Build history of the part. All positions in model axes, mm. Give positions to 0.01 mm unless a question says otherwise; leave off trailing zeros. Order: outer loops, then holes, each group sorted by start corner. A loop starts at its lowest first (then second) coordinate and runs counter-clockwise, first axis right, second up. Notation, with made-up numbers: M 9,29.25 L 36,29.25 A16 ccw 36,47.25 Z; hole C 19.5,31 d4. An arc over 180 degrees is marked long. Answer as CSV lines item,"result".
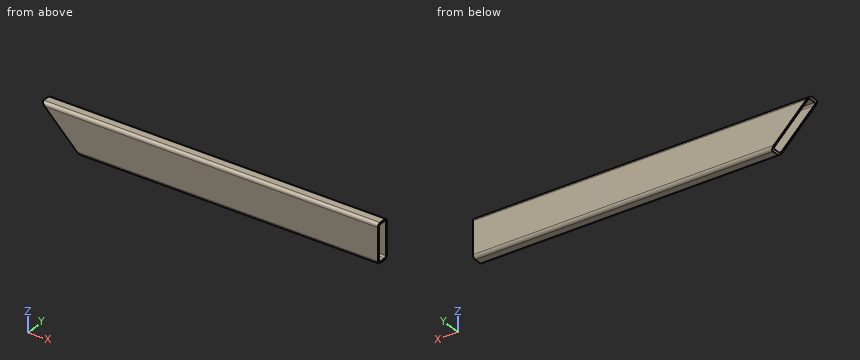
from build123d import *

# Parameters (mm, degrees)
SKETCH1_W           = 76.2
SKETCH1_H           = 25.4
BOSS_EXTRUDE1_DEPTH = 660.4
FILLET1_R           = 6.35
SHELL1_T            = -3.175
CUT_EXTRUDE1_DEPTH  = 25.4


with BuildPart() as part:
    # Sketch1 → Boss-Extrude1 (new body)
    with BuildSketch(Plane(origin=(0, 0, 0), x_dir=(0, 0, -1), z_dir=(1, 0, 0))):
        with Locations((38.1, 12.7)):
            Rectangle(SKETCH1_W, SKETCH1_H)
    extrude(amount=BOSS_EXTRUDE1_DEPTH)

    # Fillet1
    fillet1_edges = [part.edges().sort_by_distance(p)[0] for p in [
        (330.2, 25.4, 0),
        (330.2, 25.4, -76.2),
        (330.2, 0, -76.2),
        (330.2, 0, 0),
    ]]
    fillet(fillet1_edges, radius=FILLET1_R)

    # Shell1
    shell1_openings = [part.faces().sort_by_distance(p)[0] for p in [
        (660.4, 12.7, -38.1),
        (0, 12.7, -38.1),
    ]]
    offset(amount=SHELL1_T, openings=shell1_openings, kind=Kind.INTERSECTION)

    # Sketch2 → Cut-Extrude1 (cut)
    with BuildSketch(Plane(origin=(0, 25.4, 0), x_dir=(1, 0, 0), z_dir=(0, 1, 0))):
        Polygon((0, 0), (76.2, 76.2), (0, 76.2), align=None)
    extrude(amount=-CUT_EXTRUDE1_DEPTH, mode=Mode.SUBTRACT)


solid = part.part
Item 1: Band-saw the part on A-A (y = 13.5). Give the cut face in (x, z) (3 decimals).
Geometry says:
outline,"M 0,0 L 3.175,-3.175 L 660.4,-3.175 L 660.4,0 Z; M 73.025,-73.025 L 76.2,-76.2 L 660.4,-76.2 L 660.4,-73.025 Z"
Item 2: Band-saw the part on C-C (x = 246.5). Give the cut face in (y, z) (3 decimals).
Geometry says:
outline,"M 0,-69.85 A6.35 ccw 6.35,-76.2 L 19.05,-76.2 A6.35 ccw 25.4,-69.85 L 25.4,-6.35 A6.35 ccw 19.05,0 L 6.35,0 A6.35 ccw 0,-6.35 Z; hole M 3.175,-69.85 A3.175 ccw 6.35,-73.025 L 19.05,-73.025 A3.175 ccw 22.225,-69.85 L 22.225,-6.35 A3.175 ccw 19.05,-3.175 L 6.35,-3.175 A3.175 ccw 3.175,-6.35 Z"
Item 3: Drop flat-ended pins along their axis: pin 1 (8 mm diameter, centred on y = 4, z = -26, fed in from -X); pin 2 (1.5 mm diameter, centred on y = 5.5, z = -20.5, fed in from -X); pin 3 (10 mm diameter, centred on x = 76, y = 12, fed in from -Z). Give the stop position or say it passes through.
Geometry says:
pin 1,"stops at x = 22.09"
pin 2,"passes through"
pin 3,"stops at z = -76.2"
Item 4: Probe line 1 along Z through (x, y) = (292.5, 12.5) (3 decimals); line 2 along Z through (x, y) = (288.5, 19.75); line 3 along Y through (x, z) = (82, -15) (3 decimals). List the from-to ranges inside material, lowest first. Write a range as from..to.
Geometry says:
line 1,"z = -76.2..-73.025, -3.175..0"
line 2,"z = -76.16..-72.95, -3.25..-0.04"
line 3,"y = 0..3.175, 22.225..25.4"
Item 5: Band-saw the part on B-B (z = -47.5). Give the cut face in (x, y) (3 decimals).
Geometry says:
outline,"M 47.5,0 L 660.4,0 L 660.4,3.175 L 47.5,3.175 Z; M 47.5,22.225 L 660.4,22.225 L 660.4,25.4 L 47.5,25.4 Z"
